```python
from build123d import *

# Parameters (mm, degrees)
F0_R     = 39.497
F1_DEPTH = 91.186
F2_R     = 39.497
F2_R_2   = 37.465
F3_DEPTH = 56.134
F4_R     = 37.465
F4_R_2   = 32.893
F5_DEPTH = 25.4
F6_R     = 29.972
F7_DEPTH = 21.082
F9_DEPTH = 17.78


# Not quite as in the source:
# - a fillet or chamfer that OpenCascade refuses, or shapes differently, is made with other operations: its cross-section is extruded or revolved along the edge and cut away or added


with BuildPart() as f1:
    # F0 (on Front) → F1 (new body)
    with BuildSketch(Plane.XZ):
        Circle(F0_R)
    extrude(amount=F1_DEPTH)

    # F2 (on face) → F3 (cut)
    with BuildSketch(Plane.XZ.offset(91.186)):
        Circle(F2_R)
        Circle(F2_R_2, mode=Mode.SUBTRACT)
    extrude(amount=-F3_DEPTH, mode=Mode.SUBTRACT)

    # F4 (on face) → F5 (cut)
    with BuildSketch(Plane.XZ.offset(91.186)):
        Circle(F4_R)
        Circle(F4_R_2, mode=Mode.SUBTRACT)
        Circle(F4_R_2)
    extrude(amount=-F5_DEPTH, mode=Mode.SUBTRACT)

    # F6 (on face) → F7 (join)
    with BuildSketch(Plane.XZ.offset(65.786)):
        Circle(F6_R)
    extrude(amount=F7_DEPTH)

    # F8 (on face) → F9 (cut)
    with BuildSketch(Plane(origin=(0, 0, 0), x_dir=(-1, 0, 0), z_dir=(0, 1, 0))):
        with BuildLine():
            ThreePointArc((0, 23.3172), (1.113551759, 23.778448241), (1.5748, 24.892))
            ThreePointArc((1.5748, 24.892), (1.113551759, 26.005551759), (0, 26.4668))
            ThreePointArc((0, 26.4668), (-1.5748, 24.892), (0, 23.3172))
        make_face()
        with BuildLine():
            ThreePointArc((26.4668, 0), (24.892, 1.5748), (23.3172, 0))
            ThreePointArc((23.3172, 0), (24.892, -1.5748), (26.4668, 0))
        make_face()
        with BuildLine():
            ThreePointArc((1.5748, -24.892), (1.113551759, -23.778448241), (0, -23.3172))
            ThreePointArc((0, -23.3172), (-1.5748, -24.892), (0, -26.4668))
            ThreePointArc((0, -26.4668), (1.113551759, -26.005551759), (1.5748, -24.892))
        make_face()
        with BuildLine():
            ThreePointArc((-26.4668, 0), (-24.892, -1.5748), (-23.3172, 0))
            ThreePointArc((-23.3172, 0), (-24.892, 1.5748), (-26.4668, 0))
        make_face()
    extrude(amount=-F9_DEPTH, mode=Mode.SUBTRACT)

    # F10: fillet of radius 5.08 on 3 edges, made by hand

    # F10_s1 → F10_t2 (revolve, cut)
    with BuildSketch(Plane.XY):
        with BuildLine():
            ThreePointArc((37.465, -60.706), (35.9771024484, -64.2981024484), (32.385, -65.786))
            Line((32.385, -65.786), (37.465, -65.786))
            Line((37.465, -65.786), (37.465, -60.706))
        make_face()
    revolve(axis=Axis((0, -65.786, 0), (0, -1, 0)), mode=Mode.SUBTRACT)

    # F10_s3 → F10_t4 (revolve, cut)
    with BuildSketch(Plane.XY):
        with BuildLine():
            ThreePointArc((39.497, -30.988), (38.9606901303, -33.2598450651), (37.465, -35.052))
            Line((37.465, -35.052), (39.497, -35.052))
            Line((39.497, -35.052), (39.497, -30.988))
        make_face()
    revolve(axis=Axis((0, -35.052, 0), (0, -1, 0)), mode=Mode.SUBTRACT)

    # F10_s5 → F10_t6 (revolve, cut)
    with BuildSketch(Plane.XY):
        with BuildLine():
            ThreePointArc((29.972, -81.788), (28.4841024484, -85.3801024484), (24.892, -86.868))
            Line((24.892, -86.868), (29.972, -86.868))
            Line((29.972, -86.868), (29.972, -81.788))
        make_face()
    revolve(axis=Axis((0, -86.868, 0), (0, -1, 0)), mode=Mode.SUBTRACT)


solid = f1.part
```
Geometry: final body of the model. Coordinates: model frame, mm. A direction names the side the tool comes from. Give positions to 0.01 mm unless a question says otherwise; leave off trailing zeros. Loops run counter-clockwise (first coordinate to the right, second up) from the corner with the lowest first, then second, coordinate; pieces in that order, holes last. Notation, with made-up numbers: (-7, 20) - (27, 20) arc R15 cw to (27, 36) - close; hole circle Ø8 at (28.25, -23). An arc over 180 degrees is marked (long way). Answer as CSV lines item,"result". Start each with the question number.
(1) Ray query, line 1 along Y through (x, z) = (28, 14.5); line 2 along X through (y, z) = (-35, 2.5); line 3 along Y through (x, z) = (-7, 24). Return the intervals inside material, ascending. Write a range as [from, to].
(2) Reachability of faces 4 (the face through (9, -65.786, -29)), 5 (the face through (-31.343, -15.277, -24.033)), 6 (the face through (26.465, -8.766, 0.069)) from +Z, -Z, +X, -X, +Y, -Y: full face, straight path, thin tool, end or side. Return the list, or none.
(3) Mould query, pull axis Z, two halves, no side actions, for faces 1 (the face through (0, -17.78, -25)), 2 (the face through (-1, 0, 1)), 3 (the face through (-3.902, -73.675, 29.717)). Classes: +Z half, -Z half, draft (parallel to the pull), parting line (faces both ways), or undercut.
(4) Section query B-B (y = -47). Output: boundary loops of the cut face in (x, z) (3 decimals).
(5) Section query A-A (z = 0). Output: boundary loops of the cut face in (x, y) (3 decimals).
(6) Pin query (flat end, axial travel): P1, Ø10, axis at y = -41, z = -10.5, coming from the +X side; P2, Ø5, axis at x = 5.5, y = -75, coming from the +Z side; P3, Ø2, axis at y = -24, z = 13.5, coming from the +X side. Return the tip coordinate at first contact, or that it passes through.
Worked answers:
1,line 1,"y = [-65.79, 0]"
1,line 2,"x = [-37.45, 37.45]"
1,line 3,"y = [-86.87, 0]"
2,face 4,"-Y"
2,face 5,"+Y, -Y"
2,face 6,"+Y"
3,face 1,"undercut"
3,face 2,"draft"
3,face 3,"parting line"
4,outline,"circle Ø74.93 at (0, 0)"
5,outline,"(-39.497, -30.988) arc R5.08 ccw to (-37.465, -35.052) - (-37.465, -60.706) arc R5.08 ccw to (-32.385, -65.786) - (-29.972, -65.786) - (-29.972, -81.788) arc R5.08 ccw to (-24.892, -86.868) - (24.892, -86.868) arc R5.08 ccw to (29.972, -81.788) - (29.972, -65.786) - (32.385, -65.786) arc R5.08 ccw to (37.465, -60.706) - (37.465, -35.052) arc R5.08 ccw to (39.497, -30.988) - (39.497, 0) - (26.467, 0) - (26.467, -17.78) - (23.317, -17.78) - (23.317, 0) - (-23.317, 0) - (-23.317, -17.78) - (-26.467, -17.78) - (-26.467, 0) - (-39.497, 0) - close"
6,P1,"stops at x = 37.06"
6,P2,"stops at z = 29.82"
6,P3,"stops at x = 37.47"
